Model file for the job. Use its own axes, mm. Round coordinates to 2 decimals unless told otherwise and drop trailing zeros. Order: outer loops, then holes, each group sorted by start corner. A loop starts at its lowest first (then second) coordinate and runs counter-clockwise, first axis right, second up. Notation, with made-up numbers: (41.25, -26) - (90.25, -26) arc R22 cw to (90.25, -16) - close; hole circle Ø8 at (8.25, 70.25). An arc over 180 degrees is marked (long way). Answer as CSV lines item,"result". Start each with the question number.
1. Wall check: line 1 along Z through (x, y) = (82.5, 1.5); line 2 along X through (y, z) = (2.05, -90); line 3 along X through (y, z) = (2.05, -48). Give the ranges that are in metal, low to high. Write a range as [from, to].
2. Band-saw the part on C-C on z = 15. List the corners of the cut face in (x, y), then the cut area to 3 significant figures.
3. Band-saw the part on B-B on x = 75. List the corners of the cut face in (y, z), then the cut area to 3 significant figures.
4. Pull direction Z, two halves, no side cores. Call faces 1 (the face through (68.63, 1.48, 1.74)), 2 (the face through (1.7, 1.5, -78.6)), 3 (the face through (28, 0, -2)): released by +Z, released by -Z, zero draft, split by the parting line, or undercut.
5. Band-saw the part on A-A on y = 0.65. List the corners of the cut face in (x, z), then the cut area to 3 significant figures.
6. Pin check, flat tips, straight feed: pin 1 Ø1.5 at (y, z) = (1.5, 5.5) entering from +X; pin 2 Ø0.9 at (x, y) = (-3.5, 2) entering from +Z; pin 3 Ø1.5 at (y, z) = (2, -17) entering from -X. Stop position of each tip, or through.
7. Band-saw the part on D-D on z = -68. List the corners of the cut face in (x, y), then the cut area to 3 significant figures.
```python
from build123d import *

# Parameters (mm, degrees)
SKETCH4_W           = 50
SKETCH4_H           = 120
BOSS_EXTRUDE1_DEPTH = 3


with BuildPart() as part:
    # Sketch4 → Boss-Extrude1 (new body)
    with BuildSketch(Plane(origin=(0, 0, 0), x_dir=(1, 0, 0), z_dir=(0, 1, 0))):
        with BuildLine():
            ThreePointArc((-106.129032258, 127.282693525), (-128.800946783, 127.363498456), (-125.655359293, 104.910714286))
            ThreePointArc((-125.655359293, 104.910714286), (-68.616686738, 0), (-125.655359293, -104.910714286))
            ThreePointArc((-125.655359293, -104.910714286), (-128.800946783, -127.363498456), (-106.129032258, -127.282693525))
            ThreePointArc((-106.129032258, -127.282693525), (0, -78.587833096), (106.129032258, -127.282693525))
            ThreePointArc((106.129032258, -127.282693525), (128.800946783, -127.363498456), (125.655359293, -104.910714286))
            ThreePointArc((125.655359293, -104.910714286), (68.616686738, 0), (125.655359293, 104.910714286))
            ThreePointArc((125.655359293, 104.910714286), (128.800946783, 127.363498456), (106.129032258, 127.282693525))
            ThreePointArc((106.129032258, 127.282693525), (0, 78.587833096), (-106.129032258, 127.282693525))
        make_face()
        Rectangle(SKETCH4_W, SKETCH4_H, mode=Mode.SUBTRACT)
    extrude(amount=BOSS_EXTRUDE1_DEPTH)


solid = part.part
```
Reply:
1,line 1,"z = [-105.48, -57.25], [57.25, 105.48]"
1,line 2,"x = [-106.87, -55.36], [55.36, 106.87]"
1,line 3,"x = [-78.2, -25], [25, 78.2]"
2,outline,"(-69.52, 0) - (-25, 0) - (-25, 3) - (-69.52, 3) - close; (25, 0) - (69.52, 0) - (69.52, 3) - (25, 3) - close"
2,area,"267 mm2"
3,outline,"(0, -100.37) - (3, -100.37) - (3, -39.43) - (0, -39.43) - close; (0, 39.43) - (3, 39.43) - (3, 100.37) - (0, 100.37) - close"
3,area,"366 mm2"
4,face 1,"undercut"
4,face 2,"released by -Z"
4,face 3,"zero draft"
5,outline,"(-125.66, -104.91) arc R15 ccw (long way) to (-106.13, -127.28) arc R140 cw to (106.13, -127.28) arc R15 ccw (long way) to (125.66, -104.91) arc R125 cw to (125.66, 104.91) arc R15 ccw (long way) to (106.13, 127.28) arc R140 cw to (-106.13, 127.28) arc R15 ccw (long way) to (-125.66, 104.91) arc R125 cw to start; hole (-25, -60) - (25, -60) - (25, 60) - (-25, 60) - close"
5,area,"27,600 mm2"
6,pin 1,"stops at x = 68.77"
6,pin 2,"stops at z = 78.64"
6,pin 3,"stops at x = -69.88"
7,outline,"(-88.73, 0) - (88.73, 0) - (88.73, 3) - (-88.73, 3) - close"
7,area,"532 mm2"
